from build123d import *

# Parameters (mm, degrees)
F0_R     = 7.5
F1_DEPTH = 7.5
F2_R     = 2.5
F3_DEPTH = 7
F4_R     = 2.5
F5_DEPTH = 4
F6_R     = 0.875
F7_DEPTH = 4


with BuildPart() as f1:
    # F0 (on Right) → F1 (new body, symmetric)
    with BuildSketch(Plane.YZ):
        Circle(F0_R)
    extrude(amount=F1_DEPTH, both=True)

    # F2 (on Front) → F3 (join, symmetric)
    with BuildSketch(Plane.XZ):
        with Locations((7.5, 0)):
            Circle(F2_R)
    extrude(amount=F3_DEPTH, both=True)

    # F4 (on Front) → F5 (cut, symmetric)
    with BuildSketch(Plane.XZ):
        with Locations((7.5, 0)):
            Circle(F4_R)
    extrude(amount=F5_DEPTH, both=True, mode=Mode.SUBTRACT)

    # F6 (on Front) → F7 (join, symmetric)
    with BuildSketch(Plane.XZ):
        with Locations((7.5, 0)):
            Circle(F6_R)
    extrude(amount=F7_DEPTH, both=True)


solid = f1.part
Could you check a few things on this model? Use its own coordinates, in mm. A direction names the side the tool comes from. Coordinates: 2 decimals unless noted, no trailing zeros. Write each loop counter-clockwise with the first axis right and the second up, starting at its lowest first coordinate (ties: lowest second). Pieces come first, ordered by that corner, then holes. Notation, with made-up numbers: (79, 3.25) - (126, 3.25) arc R8 cw to (126, 16.25) - close; hole circle Ø1 at (13.5, -31). An arc over 180 degrees is marked (long way). Put each result on its own line as item: value. Start each with the question number.
Q1. I want a section at D-D on y = 4.5. Write out the boundary of the cut face in (x, z), plus the area to 3 significant figures.
Q2. Thinking about a two-plate mould opening in Z: for faces 4 (the cylindrical face through (10, -6, 0)), 5 (the flat face through (8, 7, 0)), 6 (the cylindrical face through (5, 0, 0)), which applies, pulls with the +Z half, pulls with the -Z half, needs draft (parallel to the pull), parting line crosses it, or undercut?
Q3. Which directions (+Z, -Z, +X, -X, +Y, -Y) give clear straight access to the entire face, cutting with the end or side of a thin tool? Please do faces 1 (the cylindrical face through (10, 5, 0)), 2 (the flat face through (7, 4, -1)), 3 (the flat face through (8, -7, 0)).
Q4. I want a section at C-C on x = 8.75. Write out the boundary of the cut face in (y, z).
Q5. I'm going to push flat-ended pins straight in: P1, Ø1.3, axis at x = 8.5, z = -0.5, coming from the +Y side; P2, Ø1.5, axis at y = -2, z = -0.5, coming from the +X side (3 decimals); P3, Ø4, axis at x = -2, y = 3, coming from the +Z side. Where does each tip first touch, or does it pass through?
Q6. I want a section at A-A on y = 0. Write out the boundary of the cut face in (x, z) (3 decimals).
Q7. Please list where these lines run through material, in increasing order: L1, parallel to Y at x = 8.5, z = 1.75; L2, parallel to X at y = 0.25, z = 5.5; L3, parallel to Y at x = 7.25, z = -1.25.
Q8. I want a section at B-B on z = 0. Write out the boundary of the cut face in (x, y) (3 decimals).
Checks:
1. outline: (-7.5, -6) - (7.5, -6) - (7.5, -2.5) arc R2.5 ccw to (7.5, 2.5) - (7.5, 6) - (-7.5, 6) - close
1. area: 190 mm²
2. face 4: parting line crosses it
2. face 5: needs draft
2. face 6: undercut
3. face 1: +X, +Y, -Y
3. face 2: none
3. face 3: +Z, -Z, +X, -Y
4. outline: (-7, -2.17) - (-4, -2.17) - (-4, 2.17) - (-7, 2.17) - close; (4, -2.17) - (7, -2.17) - (7, 2.17) - (4, 2.17) - close
5. P1: y = 7
5. P2: x = 8.375
5. P3: z = 7.43
6. outline: (-7.5, -7.5) - (7.5, -7.5) - (7.5, -2.5) arc R2.5 cw to (7.5, 2.5) - (7.5, 7.5) - (-7.5, 7.5) - close; circle Ø1.75 at (7.5, 0)
7. L1: -7 to -4, 4 to 7
7. L2: -7.5 to 7.5
7. L3: -7.4 to -4, 4 to 7.4
8. outline: (-7.5, -7.5) - (7.5, -7.5) - (7.5, -7) - (10, -7) - (10, -4) - (8.375, -4) - (8.375, 4) - (10, 4) - (10, 7) - (7.5, 7) - (7.5, 7.5) - (-7.5, 7.5) - close; hole (5, -4) - (6.625, -4) - (6.625, 4) - (5, 4) - close
